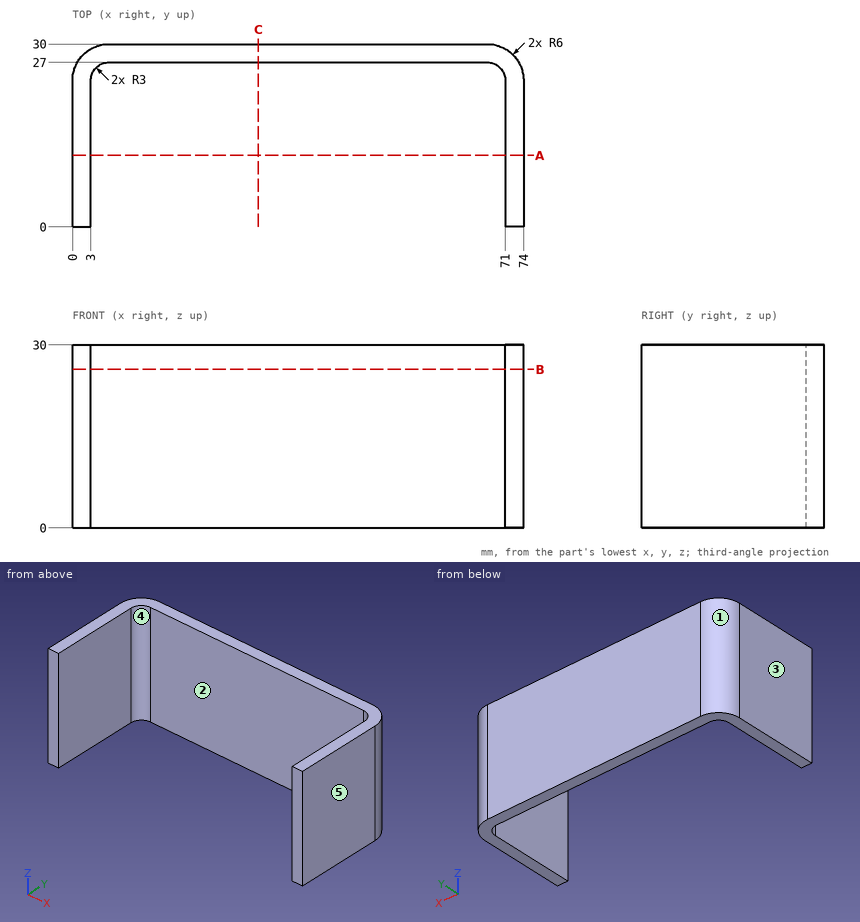
Drawing for the job (mm, zero at the part's lowest x, y, z). A direction names the side the tool comes from. Coordinates: 2 decimals unless noted, no trailing zeros. Order: outer loops, then holes, each group sorted by start corner. A loop starts at its lowest first (then second) coordinate and runs counter-clockwise, first axis right, second up. Notation, with made-up numbers: (38, 70) -> (90, 70) arc R18 ccw to (90, 96) -> close; hole circle Ø2 at (31.5, -40). An arc over 180 degrees is marked (long way). Return JSON: item names as keys, results as strings.
Item 1: Slice it at A-A (y = 11.75). Write the cut outline in (x, z), then the cut area to 3 significant figures.
Model answer:
{"outline": "(0, 0) -> (3, 0) -> (3, 30) -> (0, 30) -> close; (71, 0) -> (74, 0) -> (74, 30) -> (71, 30) -> close", "area": "180 mm²"}
Item 2: Slice it at C-C (x = 30.5). Write the cut outline in (y, z).
Model answer:
{"outline": "(27, 0) -> (30, 0) -> (30, 30) -> (27, 30) -> close"}
Item 3: Slice it at B-B (z = 26). Write the cut outline in (x, y), then the cut area to 3 significant figures.
Model answer:
{"outline": "(0, 0) -> (3, 0) -> (3, 24) arc R3 cw to (6, 27) -> (68, 27) arc R3 cw to (71, 24) -> (71, 0) -> (74, 0) -> (74, 24) arc R6 ccw to (68, 30) -> (6, 30) arc R6 ccw to (0, 24) -> close", "area": "372 mm²"}
Item 4: 3-axis set-ups, long thin cutter, end or side, ignore diameter. For the marked faces 1 and 2: which of +Z, -Z, +X, -X, +Y, -Y reach the whole face in a straight line?
Model answer:
{"face 1": "+Z, -Z, -X, +Y", "face 2": "+Z, -Z, -Y"}
Item 5: Mould opens along X. For the marked faces 3, 4 and 5 say: pulls with the +X half, pulls with the -X half, needs draft (parallel to the pull), parting line crosses it, or undercut.
Model answer:
{"face 3": "pulls with the -X half", "face 4": "undercut", "face 5": "pulls with the +X half"}
Item 6: Pin check, flat tips, straight feed: P1, Ø2, axis at x = 10.5, z = 14, coming from the -Y side; P2, Ø3, axis at y = 26, z = 27, coming from the +X side; P3, Ø8, axis at y = 21, z = 16, coming from the -X side. Stop position of each tip, or through.
Model answer:
{"P1": "stops at y = 27", "P2": "stops at x = 73.98", "P3": "stops at x = 0"}
Item 7: Wall check: line 1 along X through (y, z) = (8, 12.5); line 2 along Y through (x, z) = (11, 21.75); line 3 along X through (y, z) = (28, 15). Give the ranges that are in metal, low to high. Write a range as from..to.
Model answer:
{"line 1": "x = 0..3, 71..74", "line 2": "y = 27..30", "line 3": "x = 1.53..72.47"}
